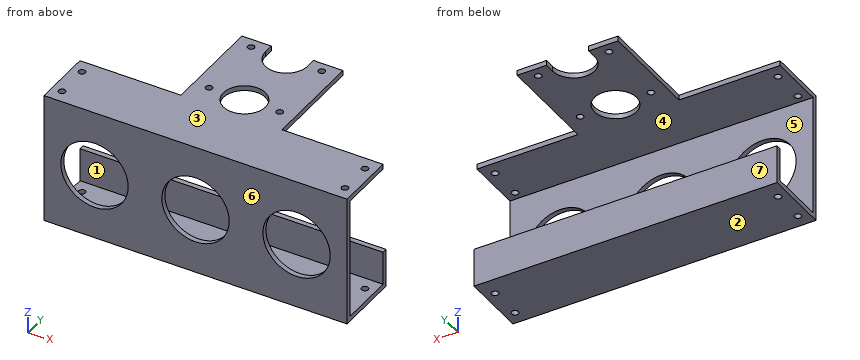
```python
from build123d import *

# Parameters (mm, degrees)
F0_W      = 30
F0_H      = 48.5
F1_DEPTH  = 1.5
F2_W      = 30
F2_H      = 1.5
F3_DEPTH  = 37.5
F4_W      = 30
F4_H      = 1.5
F5_DEPTH  = 18
F6_W      = 30
F6_H      = 1.5
F7_DEPTH  = 10
F9_DEPTH  = 30
F11_R     = 1
F11_R_2   = 6.25
F12_DEPTH = 1.5
F13_R     = 1
F14_DEPTH = 1.5
F15_R     = 10
F16_DEPTH = 1.5


with BuildPart() as f1:
    # F0 (on Top) → F1 (new body)
    with BuildSketch(Plane.XY):
        Rectangle(F0_W, F0_H)
    extrude(amount=F1_DEPTH)

    # F2 (on face) → F3 (join)
    with BuildSketch(Plane(origin=(0, 0, 0), x_dir=(1, 0, 0), z_dir=(0, 0, -1))):
        with Locations((0, 23.5)):
            Rectangle(F2_W, F2_H)
    extrude(amount=F3_DEPTH)

    # F4 (on face) → F5 (join)
    with BuildSketch(Plane(origin=(0, -22.75, 0), x_dir=(-1, 0, 0), z_dir=(0, 1, 0))):
        with Locations((0, -36.75)):
            Rectangle(F4_W, F4_H)
    extrude(amount=F5_DEPTH)

    # F6 (on face) → F7 (join)
    with BuildSketch(Plane.XY.offset(-36)):
        with Locations((0, -5.5)):
            Rectangle(F6_W, F6_H)
    extrude(amount=F7_DEPTH)

    # F8 (on face) → F9 (join)
    with BuildSketch(Plane.YZ.offset(15)):
        Polygon((-22.75, 1.5), (-24.25, 1.5), (-24.25, -37.5), (-22.75, -37.5), (-6.25, -37.5), (-4.75, -37.5), (-4.75, -26), (-6.25, -26), (-6.25, -36), (-22.75, -36), (-22.75, 0), (-6.25, 0), (-6.25, 1.5), align=None)
    extrude(amount=F9_DEPTH)

    # F10: F1 across plane


with BuildPart() as f1_1:
    add(f1.part)
    add(f1.part.mirror(Plane.YZ))

    # F11 (on face) → F12 (cut, through all)
    with BuildSketch(Plane.XY.offset(1.5)):
        with Locations((10.5, 21.25)):
            Circle(F11_R)
        with Locations((10.5, 0.25)):
            Circle(F11_R)
        with BuildLine():
            Line((-6.25, 24.25), (-6.25, 21.25))
            ThreePointArc((-6.25, 21.25), (0, 15), (6.25, 21.25))
            Line((6.25, 21.25), (6.25, 24.25))
            Line((6.25, 24.25), (-6.25, 24.25))
        make_face()
        with Locations((-10.5, 21.25)):
            Circle(F11_R)
        with Locations((-10.5, 0.25)):
            Circle(F11_R)
        with Locations((0, 0.25)):
            Circle(F11_R_2)
        with Locations((-42, -10.25)):
            Circle(F11_R)
        with Locations((-42, -20.25)):
            Circle(F11_R)
        with Locations((42, -10.25)):
            Circle(F11_R)
        with Locations((42, -20.25)):
            Circle(F11_R)
    extrude(amount=-F12_DEPTH, mode=Mode.SUBTRACT)

    # F13 (on face) → F14 (cut, through all)
    with BuildSketch(Plane.XY.offset(-36)):
        with Locations((-42, -10.25)):
            Circle(F13_R)
        with Locations((-42, -20.25)):
            Circle(F13_R)
        with Locations((42, -10.25)):
            Circle(F13_R)
        with Locations((42, -20.25)):
            Circle(F13_R)
    extrude(amount=-F14_DEPTH, mode=Mode.SUBTRACT)

    # F15 (on face) → F16 (cut, through all)
    with BuildSketch(Plane.XZ.offset(24.25)):
        with Locations((0, -18)):
            Circle(F15_R)
        with Locations((-30, -18)):
            Circle(F15_R)
        with Locations((30, -18)):
            Circle(F15_R)
    extrude(amount=-F16_DEPTH, mode=Mode.SUBTRACT)


solid = f1_1.part
```
Geometry: final body of the model. Coordinates: model frame, mm. Face numbers are marked on the shaded views. A direction names the side the tool comes from. Coordinates: 2 decimals unless noted, no trailing zeros. Loops run counter-clockwise (first coordinate to the right, second up) from the corner with the lowest first, then second, coordinate; pieces in that order, holes last. Notation, with made-up numbers: (65.5, 20.5) -> (96.5, 20.5) arc R24 ccw to (96.5, 48.5) -> close; hole circle Ø2 at (84.25, -15.75). An arc over 180 degrees is marked (long way). Use a Markdown table: item, result. Add a question column.
(1) Section query B-B, the plane x = -22. Return loops of the section in (y, z).
(2) Line query: line 1 along Y through (x, z) = (-42, -36.9); line 2 along Z through (x, y) = (-26.5, -21); line 3 along Y through (x, z) = (-42, 1.1). Output: solid intervals per line, ascending.
(3) Access query for the marked faces 4, 5, 6 and 7. Directions: +Z, -Z, +X, -X, +Y, -Y. A direction counts if a zero-diameter tool reaches every point of the face in a straight line with its end or side. Return the directions, or none.
(4) Section query A-A, the plane z = -29.5. Return loops of the section in (x, y).
(5) Pin query (flat end, axial travel): pin 1 Ø1.8 at (x, y) = (-42, -10.25) entering from +Z. Return the tip coordinate at first contact, or that it passes through.
(6) Section query C-C, the plane y = 0.25. Return loops of the section in (x, z), plus the area to 4 significant figures.
(7) Section query D-D, the plane x = 0. Return loops of the section in (y, z).
(8) Mould query, pull axis Z, two halves, no side actions, for the marked faces 1, 2 and 3. Classes: pulls with the +Z half, pulls with the -Z half, needs draft (parallel to the pull), parting line crosses it, or undercut.
Answer:
| question | item | result |
|---|---|---|
| 1 | outline | (-24.25, -37.5) -> (-4.75, -37.5) -> (-4.75, -26) -> (-6.25, -26) -> (-6.25, -36) -> (-22.75, -36) -> (-22.75, -24) -> (-24.25, -24) -> close; (-24.25, -12) -> (-22.75, -12) -> (-22.75, 0) -> (-6.25, 0) -> (-6.25, 1.5) -> (-24.25, 1.5) -> close |
| 2 | line 1 | y = -24.25 to -21.25, -19.25 to -11.25, -9.25 to -4.75 |
| 2 | line 2 | z = -37.5 to -36, 0 to 1.5 |
| 2 | line 3 | y = -24.25 to -21.25, -19.25 to -11.25, -9.25 to -6.25 |
| 3 | face 4 | +X, -X, +Y |
| 3 | face 5 | +X, -X |
| 3 | face 6 | +Z, -Z, +X, -X, -Y |
| 3 | face 7 | -Z, +X, -X, +Y |
| 4 | outline | (-45, -24.25) -> (45, -24.25) -> (45, -22.75) -> (-45, -22.75) -> close; (-45, -6.25) -> (45, -6.25) -> (45, -4.75) -> (-45, -4.75) -> close |
| 5 | pin 1 | passes through |
| 6 | outline | (-15, 0) -> (-11.5, 0) -> (-11.5, 1.5) -> (-15, 1.5) -> close; (-9.5, 0) -> (-6.25, 0) -> (-6.25, 1.5) -> (-9.5, 1.5) -> close; (6.25, 0) -> (9.5, 0) -> (9.5, 1.5) -> (6.25, 1.5) -> close; (11.5, 0) -> (15, 0) -> (15, 1.5) -> (11.5, 1.5) -> close |
| 6 | area | 20.25 mm^2 |
| 7 | outline | (-24.25, -37.5) -> (-4.75, -37.5) -> (-4.75, -26) -> (-6.25, -26) -> (-6.25, -36) -> (-22.75, -36) -> (-22.75, -28) -> (-24.25, -28) -> close; (-24.25, -8) -> (-22.75, -8) -> (-22.75, 0) -> (-6, 0) -> (-6, 1.5) -> (-24.25, 1.5) -> close; (6.5, 0) -> (15, 0) -> (15, 1.5) -> (6.5, 1.5) -> close |
| 8 | face 1 | undercut |
| 8 | face 2 | pulls with the -Z half |
| 8 | face 3 | pulls with the +Z half |
